```python
from build123d import *

# Parameters (mm, degrees)
F1_DEPTH = 5


with BuildPart() as f1:
    # F0 (on Top) → F1 (new body)
    with BuildSketch(Plane.XY):
        with BuildLine():
            Line((-2.80428, 11.038499), (-2.80428, 14.735536))
            ThreePointArc((-2.80428, 14.735536), (-14.933738, -1.408361), (0, -15))
            Line((0, -15), (0, -29.789679))
            Line((0, -29.789679), (4.604714, -29.789679))
            Line((4.604714, -29.789679), (4.604714, -15))
            Line((4.604714, -15), (4.239221, -13.388641))
            ThreePointArc((4.239221, -13.388641), (-8.082837, -3.712616), (-2.80428, 11.038499))
        make_face()
        with BuildLine():
            Line((0, 5.920346), (0, 15))
            ThreePointArc((0, 15), (-1.408361, 14.933738), (-2.80428, 14.735536))
            Line((-2.80428, 14.735536), (-2.80428, 11.038499))
            Line((-2.80428, 11.038499), (-2.80428, 5.920346))
            Line((-2.80428, 5.920346), (0, 5.920346))
        make_face()
    extrude(amount=F1_DEPTH)


solid = f1.part
```
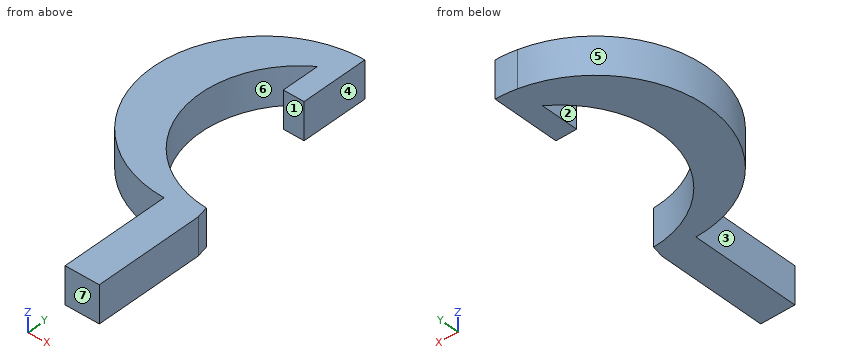
Input: part model. Units: mm. Frame: model coordinates. Face numbers are marked on the shaded views. A direction names the side the tool comes from. Give positions to 0.01 mm unless a question says otherwise; leave off trailing zeros. Order: outer loops, then holes, each group sorted by start corner. A loop starts at its lowest first (then second) coordinate and runs counter-clockwise, first axis right, second up. Notation, with made-up numbers: M 87,9.5 L 122,9.5 A29 cw 122,42.5 Z; hole C 64,57 d10. An arc over 180 degrees is marked long. Return JSON: item names as keys, results as strings.
Item 1: Cut plane A-A (z = 2.2). Return loops of the section in (x, y).
Solutions:
{"outline": "M -2.8,5.92 L 0,5.92 L 0,15 A15 ccw -2.8,14.74 A15 ccw 0,-15 L 0,-29.79 L 4.6,-29.79 L 4.6,-15 L 4.24,-13.39 A13.4 cw -2.8,11.04 Z"}
Item 2: First-contact query: P1, Ø1.5, axis at x = -4, z = 3.5, coming from the -Y side; P2, Ø1.5, axis at y = -9.5, z = 1.5, coming from the +X side; P3, Ø1.5, axis at y = 8, z = 1.5, coming from the -X side. Flat tips, straight axial feed; report the tip coordinate or a pass-through.
Solutions:
{"P1": "y = -14.64", "P2": "x = -3.84", "P3": "x = -13.13"}
Item 3: Pull-direction query (Y, two-part tool) for the marked faces 5, 6 and 7; classes: +Y half, -Y half, draft (parallel to the pull), parting line (faces both ways), or undercut.
Solutions:
{"face 5": "parting line", "face 6": "undercut", "face 7": "-Y half"}
Item 4: Ray query, probe 1 along X at (y, z) = (-19.5, 2.7); probe 2 along X at (y, z) = (9, 4.8); probe 3 along Y at (x, z) = (-4.25, 1.45). Return the intervals inside material, ascending.
Solutions:
{"probe 1": "0 to 4.6", "probe 2": "-12 to -5.14, -2.8 to 0", "probe 3": "-14.39 to -9.89, 9.89 to 14.39"}
Item 5: Access query for the marked faces 1, 2, 3 and 4. Directions: +Z, -Z, +X, -X, +Y, -Y. A direction counts if a zero-diameter tool reaches every point of the face in a straight line with its end or side. Return the directions, or none.
Solutions:
{"face 1": "+Z, -Z, +X", "face 2": "+Z, -Z", "face 3": "+Z, -Z, -X, -Y", "face 4": "+Z, -Z, +X, +Y"}
Item 6: Cut plane C-C (y = 10). Return loops of the section in (x, z).
Solutions:
{"outline": "M -11.18,0 L -4.13,0 L -4.13,5 L -11.18,5 Z; M -2.8,0 L 0,0 L 0,5 L -2.8,5 Z"}
Item 7: Cut plane D-D (y = -18). Return loops of the section in (x, z), then the cut area to 3 significant figures.
Solutions:
{"outline": "M 0,0 L 4.6,0 L 4.6,5 L 0,5 Z", "area": "23.0 mm^2"}
Item 8: Cut plane B-B (x = -6.5). Return loops of the section in (y, z).
Solutions:
{"outline": "M -13.52,0 L -7.21,0 L -7.21,5 L -13.52,5 Z; M 7.21,0 L 13.52,0 L 13.52,5 L 7.21,5 Z"}
